For this review, take the finished solid that the model builds, in its own axes (mm). A direction names the side the tool comes from. Give positions to 0.01 mm unless a question says otherwise; leave off trailing zeros. Loops run counter-clockwise (first coordinate to the right, second up) from the corner with the lowest first, then second, coordinate; pieces in that order, holes last. Notation, with made-up numbers: (-20.75, 52) - (14.25, 52) arc R15 cw to (14.25, 74) - close; hole circle Ø10 at (-13, 14). An arc over 180 degrees is marked (long way). Answer in a Markdown table with one row per item.
```python
from build123d import *

# Parameters (mm, degrees)
SKETCH1_W           = 24
SKETCH1_H           = 24
BOSS_EXTRUDE1_DEPTH = 17
CUT_EXTRUDE1_DEPTH  = 32.764760349
SKETCH3_R           = 9
BOSS_EXTRUDE2_DEPTH = 52
BOSS_EXTRUDE3_DEPTH = 16
CHAMFER1_START      = 46.9999999
CHAMFER1_OUTLINE_R  = 9
CHAMFER1_DEPTH      = 5.0000001
SKETCH5_W           = 11
SKETCH5_H           = 8
BOSS_EXTRUDE4_DEPTH = 7
SKETCH6_R           = 2.05
CUT_EXTRUDE2_DEPTH  = 6


with BuildPart() as part:
    # Sketch1 → Boss-Extrude1 (new body)
    with BuildSketch(Plane(origin=(0, 0, 0), x_dir=(1, 0, 0), z_dir=(0, 1, 0))):
        Rectangle(SKETCH1_W, SKETCH1_H)
    extrude(amount=BOSS_EXTRUDE1_DEPTH)

    # Sketch2 → Cut-Extrude1 (cut, through all)
    with BuildSketch(Plane.ZY.offset(12)):
        Polygon((-12, 17), (12, 13), (12, 17), align=None)
    extrude(amount=-CUT_EXTRUDE1_DEPTH, mode=Mode.SUBTRACT)

    # Sketch3 → Boss-Extrude2 (add)
    with BuildSketch(Plane.XZ):
        with Locations(Location((0, 0, 0), (0, 0, 270))):
            Circle(SKETCH3_R)
    extrude(amount=-BOSS_EXTRUDE2_DEPTH)

    # Sketch4 → Boss-Extrude3 (add)
    with BuildSketch(Plane(origin=(0, 52, 0), x_dir=(1, 0, 0), z_dir=(0, 1, 0))):
        with BuildLine():
            Line((-9.456572951, 0.90731914), (-9.84083402, -3.097658461))
            ThreePointArc((-9.84083402, -3.097658461), (-8.220587121, -7.800746053), (-3.608813676, -9.665090067))
            Line((-3.608813676, -9.665090067), (0.410792593, -9.491114236))
            ThreePointArc((0.410792593, -9.491114236), (6.891182028, 6.539236214), (-9.456572951, 0.90731914))
        make_face()
    extrude(amount=BOSS_EXTRUDE3_DEPTH)

    # Chamfer1: read off the stored shape, not the designer's step
    # Chamfer1 outline → Chamfer1 (add)
    with BuildSketch(Plane(origin=(0, 0, 0), x_dir=(1, 0, 0), z_dir=(0, 1, 0)).offset(CHAMFER1_START)):
        with BuildLine():
            ThreePointArc((-9.84083402, -3.097658461), (-8.220587121, -7.800746053), (-3.608813676, -9.665090067))
            Line((-3.608813676, -9.665090067), (0.410792593, -9.491114236))
            ThreePointArc((0.410792593, -9.491114236), (6.891182028, 6.539236214), (-9.456572951, 0.90731914))
            Line((-9.456572951, 0.90731914), (-9.84083402, -3.097658461))
        make_face()
        Circle(CHAMFER1_OUTLINE_R, mode=Mode.SUBTRACT)
    extrude(amount=CHAMFER1_DEPTH)

    # Chamfer1 2 outline → Chamfer1 2 (revolve, cut)
    with BuildSketch(Plane.XY):
        Polygon((11.332682454, 49.332682454), (9, 47), (11.332682454, 46.9999999), align=None)
    revolve(axis=Axis((0, 0, 0), (0, 1, 0)), mode=Mode.SUBTRACT)

    # Sketch5 → Boss-Extrude4 (add)
    with BuildSketch(Plane(origin=(0, 68, 0), x_dir=(1, 0, 0), z_dir=(0, 1, 0))):
        Rectangle(SKETCH5_W, SKETCH5_H)
    extrude(amount=BOSS_EXTRUDE4_DEPTH)

    # Sketch6 → Cut-Extrude2 (cut)
    with BuildSketch(Plane(origin=(0, 0, -12), x_dir=(-1, 0, 0), z_dir=(0, 0, -1))):
        with Locations((5, 12)):
            Circle(SKETCH6_R)
        with Locations((-5, 12)):
            Circle(SKETCH6_R)
    extrude(amount=-CUT_EXTRUDE2_DEPTH, mode=Mode.SUBTRACT)


solid = part.part
```
1. For faces 5 (the face through (7.097, 57.606, -6.315)), 6 (the face through (-5.5, 71, 0)), 7 (the face through (-9.646, 57.606, 1.067)), 8 (the face through (-5, 12, -6)), 9 (the face through (5.5, 71, 0)), list the 3-axis set-ups (+Z, -Z, +X, -X, +Y, -Y) from which the entire face can be reached by the end or side of a thin tool; tool diameter is ignored.
Values:
| item | result |
|---|---|
| face 5 | +Y |
| face 6 | +Z, -Z, -X, +Y |
| face 7 | -Z, -X, +Y |
| face 8 | -Z |
| face 9 | +Z, -Z, +X, +Y |
2. Mouldability with a two-part tool opening along Z and no side actions: class faces 1 (the face through (0, 71, -4)), 2 (the face through (-8.17, 14.14, 5.17)), 3 (the face through (-5.555, 47.124, 7.238)), 4 (the face through (0, 0, 0)) as released by +Z, released by -Z, zero draft, split by the parting line, or undercut.
Values:
| item | result |
|---|---|
| face 1 | released by -Z |
| face 2 | undercut |
| face 3 | split by the parting line |
| face 4 | zero draft |
3. We need section B-B, the plane z = 0. Give the boundary of the cut face in (x, y).
Values:
| item | result |
|---|---|
| outline | (-12, 0) - (12, 0) - (12, 15) - (9, 15) - (9, 47) - (9.5, 47.5) - (9.5, 68) - (5.5, 68) - (5.5, 75) - (-5.5, 75) - (-5.5, 68) - (-9.54, 68) - (-9.54, 47.54) - (-9, 47) - (-9, 15) - (-12, 15) - close |
4. We need section C-C, the plane y = 37. Give the boundary of the cut face in (x, z), and give its area (3 significant figures).
Values:
| item | result |
|---|---|
| outline | circle Ø18 at (0, 0) |
| area | 254 mm^2 |
5. Wall thickness on line 1 (Y direction, x = 5, z = -7.35); line 2 (Y direction, x = 5.75, z = 0); line 3 (Y direction, x = 5, z = -9.2): over which ranges is each line inside the solid? List them lowest first. Write a range as [from, to].
Values:
| item | result |
|---|---|
| line 1 | y = [0, 9.95], [14.05, 68] |
| line 2 | y = [0, 68] |
| line 3 | y = [0, 9.95], [14.05, 16.53] |
6. We need section D-D, the plane y = 62.5. Give the boundary of the cut face in (x, z).
Values:
| item | result |
|---|---|
| outline | (-9.84, 3.1) - (-9.46, -0.91) arc R9.5 ccw (long way) to (0.41, 9.49) - (-3.61, 9.67) arc R6 ccw to start |
7. We need section A-A, the plane y = 12. Give the boundary of the cut face in (x, z), and give its area (3 significant figures).
Values:
| item | result |
|---|---|
| outline | (-12, -12) - (-7.05, -12) - (-7.05, -6) - (-2.95, -6) - (-2.95, -12) - (2.95, -12) - (2.95, -6) - (7.05, -6) - (7.05, -12) - (12, -12) - (12, 12) - (-12, 12) - close |
| area | 527 mm^2 |
8. Clearance check with flat-ended pins moving along their axes: pin 1 (2 mm diameter, centred on x = -8.5, z = 5.5, fed in from +Y); pin 2 (3.5 mm diameter, centred on x = -0.5, y = 72.5, fed in from +Z); pin 3 (5 mm diameter, centred on y = 60, z = -2.5, fed in from -X). State where each tip first meets the part, or that it passes through.
Values:
| item | result |
|---|---|
| pin 1 | stops at y = 68 |
| pin 2 | stops at z = 4 |
| pin 3 | stops at x = -9.54 |
